The listing builds one solid part. Answer for the finished solid, in the listing's coordinates (mm). Face numbers are marked on the shaded views. A direction names the side the tool comes from. Coordinates: 2 decimals unless noted, no trailing zeros. Order: outer loops, then holes, each group sorted by start corner. A loop starts at its lowest first (then second) coordinate and runs counter-clockwise, first axis right, second up. Notation, with made-up numbers: (28.5, 53) -> (86.5, 53) arc R17 cw to (86.5, 63) -> close; hole circle Ø5 at (-23.5, -18). An arc over 180 degrees is marked (long way). Write item = value, one per line.
from build123d import *

# Parameters (mm, degrees)
BOSS_EXTRU_1_DEPTH             = 3.175
ESQUISSE3_R                    = 2.1
ENL_V_MAT_EXTRU_1_DEPTH        = 51.235046687
ENL_V_MAT_EXTRU_2_DEPTH        = 3.175
CONG_1_R                       = 15.24
CONG_2_R                       = 15.24
BOSS_EXTRU_3_REACH             = 51.933
BOSS_EXTRU_3_DIRECTION_2_REACH = 51.933
ENL_V_MAT_EXTRU_3_DEPTH        = 3.175
CONG_3_R                       = 2.54


with BuildPart() as part:
    # Esquisse2 → Boss.-Extru.1 (new, symmetric)
    with BuildSketch(Plane.XY):
        with BuildLine():
            Line((25.4, 0), (33.652960284, 25.4))
            ThreePointArc((33.652960284, 25.4), (28.67359617, 35.819836664), (18.013926444, 31.377032999))
            Line((18.013926444, 31.377032999), (10.16, 13.597032999))
            Line((10.16, 13.597032999), (-10.16, 13.597032999))
            Line((-10.16, 13.597032999), (-18.013926444, 31.377032999))
            ThreePointArc((-18.013926444, 31.377032999), (-28.67359617, 35.819836664), (-33.652960284, 25.4))
            Line((-33.652960284, 25.4), (-25.4, 0))
            Line((-25.4, 0), (-25.4, -12.7))
            Line((-25.4, -12.7), (25.4, -12.7))
            Line((25.4, -12.7), (25.4, 0))
        make_face()
    extrude(amount=BOSS_EXTRU_1_DEPTH, both=True)

    # Esquisse3 → Enlèv. mat.-Extru.1 (cut, through all)
    with BuildSketch(Plane.XY.offset(3.175)):
        with Locations((-25.673864308, 27.96758946)):
            Circle(ESQUISSE3_R)
    enl_v_mat_extru_1 = extrude(amount=-ENL_V_MAT_EXTRU_1_DEPTH, mode=Mode.SUBTRACT)

    # Symétrie1: Enlèv. mat.-Extru.1 across plane
    add(enl_v_mat_extru_1.mirror(Plane(origin=(0, 0, 0), x_dir=(0, 0, 1), z_dir=(1, 0, 0))), mode=Mode.SUBTRACT)

    # Esquisse4 → Enlèv. mat.-Extru.2 (cut)
    with BuildSketch(Plane.XY.offset(3.175)):
        Polygon((27.454849211, 6.324175587), (-27.454849211, 6.324175587), (-25.4, 0), (-25.4, -12.7), (25.4, -12.7), (25.4, 0), align=None)
    extrude(amount=-ENL_V_MAT_EXTRU_2_DEPTH, mode=Mode.SUBTRACT)

    # Congé1
    cong_1_edges = [part.edges().sort_by_distance(p)[0] for p in [
        (-10.16, 13.597032999, 0),
        (10.16, 13.597032999, 0),
    ]]
    fillet(cong_1_edges, radius=CONG_1_R)

    # Congé2
    cong_2_edges = [part.edges().sort_by_distance(p)[0] for p in [
        (-25.4, 0, -1.5875),
        (25.4, 0, -1.5875),
    ]]
    fillet(cong_2_edges, radius=CONG_2_R)

    # Boss.-Extru.3: up to this face of the body (flat: up to its plane)
    boss_extru_3_end = Plane(part.part.faces().sort_by_distance((-16.773966377, 26.7272166, 3.175))[0])
    # Esquisse8 → Boss.-Extru.3 (add, up to the picked face)
    with BuildSketch(Plane.XY, mode=Mode.PRIVATE) as boss_extru_3_sk1:
        with BuildLine():
            Line((-27.454849211, 6.324175587), (-26.145898692, 2.295640124))
            ThreePointArc((-26.145898692, 2.295640124), (-25.821082413, 1.143928475), (-25.587629689, -0.029717623))
            Line((-25.587629689, -0.029717623), (-34.063204565, -0.029717623))
            Line((-34.063204565, -0.029717623), (-34.063204565, 27.990180447))
            ThreePointArc((-34.063204565, 27.990180447), (-33.960008236, 26.678946761), (-33.652960284, 25.4))
            Line((-33.652960284, 25.4), (-27.454849211, 6.324175587))
        make_face()
    boss_extru_3_tool1 = split(extrude(boss_extru_3_sk1.sketch, amount=BOSS_EXTRU_3_REACH, mode=Mode.PRIVATE), bisect_by=boss_extru_3_end, keep=Keep.BOTH, mode=Mode.PRIVATE)
    boss_extru_3 = boss_extru_3_tool1.solids().sort_by(Axis((-31.181863, 8.892932, 0), (0, 0, 1)))[0]
    add(boss_extru_3)

    # Boss.-Extru.3 direction 2: up to this face of the body (flat: up to its plane)
    boss_extru_3_direction_2_end = Plane(part.part.faces().sort_by_distance((0, 8.816587411, -3.175))[0])
    # Esquisse8 → Boss.-Extru.3 direction 2 (add, up to the picked face)
    with BuildSketch(Plane.XY, mode=Mode.PRIVATE) as boss_extru_3_direction_2_sk1:
        with BuildLine():
            Line((-27.454849211, 6.324175587), (-26.145898692, 2.295640124))
            ThreePointArc((-26.145898692, 2.295640124), (-25.821082413, 1.143928475), (-25.587629689, -0.029717623))
            Line((-25.587629689, -0.029717623), (-34.063204565, -0.029717623))
            Line((-34.063204565, -0.029717623), (-34.063204565, 27.990180447))
            ThreePointArc((-34.063204565, 27.990180447), (-33.960008236, 26.678946761), (-33.652960284, 25.4))
            Line((-33.652960284, 25.4), (-27.454849211, 6.324175587))
        make_face()
    boss_extru_3_direction_2_tool1 = split(extrude(boss_extru_3_direction_2_sk1.sketch, amount=-BOSS_EXTRU_3_DIRECTION_2_REACH, mode=Mode.PRIVATE), bisect_by=boss_extru_3_direction_2_end, keep=Keep.BOTH, mode=Mode.PRIVATE)
    boss_extru_3_direction_2 = boss_extru_3_direction_2_tool1.solids().sort_by(Axis((-31.181863, 8.892932, 0), (0, 0, -1)))[0]
    add(boss_extru_3_direction_2)

    # Symétrie2: Boss.-Extru.3, Boss.-Extru.3 direction 2 across plane
    add(boss_extru_3.mirror(Plane(origin=(0, 0, 0), x_dir=(0, 0, 1), z_dir=(1, 0, 0))))
    add(boss_extru_3_direction_2.mirror(Plane(origin=(0, 0, 0), x_dir=(0, 0, 1), z_dir=(1, 0, 0))))

    # Esquisse9 → Enlèv. mat.-Extru.3 (cut)
    with BuildSketch(Plane.XY.offset(3.175)):
        with BuildLine():
            Line((-27.454849211, 6.324175587), (-26.145898692, 2.295640124))
            ThreePointArc((-26.145898692, 2.295640124), (-25.821082413, 1.143928475), (-25.587629689, -0.029717623))
            Line((-25.587629689, -0.029717623), (-34.063204565, -0.029717623))
            Line((-34.063204565, -0.029717623), (-34.063204565, 6.324175587))
            Line((-34.063204565, 6.324175587), (-27.454849211, 6.324175587))
        make_face()
    enl_v_mat_extru_3 = extrude(amount=-ENL_V_MAT_EXTRU_3_DEPTH, mode=Mode.SUBTRACT)

    # Symétrie3: Enlèv. mat.-Extru.3 across plane
    add(enl_v_mat_extru_3.mirror(Plane(origin=(0, 0, 0), x_dir=(0, 0, 1), z_dir=(1, 0, 0))), mode=Mode.SUBTRACT)

    # Congé3
    cong_3_edges = [part.edges().sort_by_distance(p)[0] for p in [
        (25.587629689, -0.029717623, -1.5875),
        (-25.587629689, -0.029717623, -1.5875),
    ]]
    fillet(cong_3_edges, radius=CONG_3_R)


solid = part.part
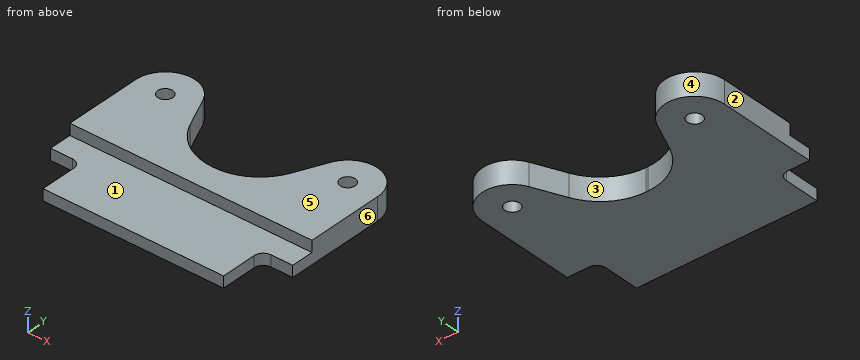
Q1. Find the intervals of material crossed by line 1 along X through (y, z) = (18, 1.5); line 2 along Z through (x, y) = (-21, -2.5) (3 decimals); line 3 along X through (y, z) = (19, 2.25), in increasing order.
The answers:
line_1 = -34.06 to -10.95, 10.95 to 34.06
line_2 = -3.175 to 0
line_3 = -34.06 to -11.87, 11.87 to 34.06
Q2. Section C-C, the plane z = 1.25 is taken. Give the vertices of the cut face in (x, y).
The answers:
outline = (-34.06, 6.32) -> (34.06, 6.32) -> (34.06, 27.99) arc R8.38 ccw to (18.01, 31.38) -> (14.17, 22.68) arc R15.24 cw to (0.23, 13.6) -> (-0.23, 13.6) arc R15.24 cw to (-14.17, 22.68) -> (-18.01, 31.38) arc R8.38 ccw to (-34.06, 27.99) -> close; hole circle Ø4.2 at (-25.67, 27.97); hole circle Ø4.2 at (25.67, 27.97)
Q3. Section D-D, the plane x = 5 is taken. Give the vertices of the cut face in (y, z) (3 decimals).
The answers:
outline = (-12.7, -3.175) -> (14.362, -3.175) -> (14.362, 3.175) -> (6.324, 3.175) -> (6.324, 0) -> (-12.7, 0) -> close
Q4. The mould has two halves that part along X. Classify the marked faces 4, 5 and 6: released by +X, released by -X, zero draft, split by the parting line, or undercut.
The answers:
face_4 = undercut
face_5 = zero draft
face_6 = released by +X
Q5. Section B-B, the plane y = 14.5 is taken. Give the vertices of the cut face in (x, z) (3 decimals).
The answers:
outline = (-34.063, -3.175) -> (-5.399, -3.175) -> (-5.399, 3.175) -> (-34.063, 3.175) -> close; (5.399, -3.175) -> (34.063, -3.175) -> (34.063, 3.175) -> (5.399, 3.175) -> close
Q6. Each of these flat-tipped pins is pushed along its axis until it touches: pin 1 Ø2.5 at (x, y) = (-25.67, 27.97) entering from -Z; pin 2 Ø3.5 at (x, z) = (-30, -1.5) entering from -Y; pin 3 Ø2.5 at (y, z) = (-8.5, -1.5) entering from -X; pin 4 Ø4 at (x, y) = (-24.5, -1) entering from +Z. Where does it stop, or does it pass through?
The answers:
pin_1 = through
pin_2 = -0.03
pin_3 = -25.4
pin_4 = 0
Q7. A tool of negligible diameter and unlimited length cuts with its end or side. For the marked faces 1, 2 and 3, from which of +Z, -Z, +X, -X, +Y, -Y can it reach the whole face along a straight path? Write none if from no direction.
The answers:
face_1 = +Z, +X, -X, -Y
face_2 = +Z, -Z, -X, +Y, -Y
face_3 = +Z, -Z, +Y
Q8. Section A-A, the plane y = 29 is taken. Give the vertices of the cut face in (x, z) (3 decimals), plus the area to 3 significant figures.
The answers:
outline = (-34.002, -3.175) -> (-27.503, -3.175) -> (-27.503, 3.175) -> (-34.002, 3.175) -> close; (-23.845, -3.175) -> (-16.964, -3.175) -> (-16.964, 3.175) -> (-23.845, 3.175) -> close; (16.964, -3.175) -> (23.845, -3.175) -> (23.845, 3.175) -> (16.964, 3.175) -> close; (27.503, -3.175) -> (34.002, -3.175) -> (34.002, 3.175) -> (27.503, 3.175) -> close
area = 170 mm2
